Work out the finished part from the listing and answer in its coordinate system (mm). A direction names the side the tool comes from. Give positions to 0.01 mm unless a question says otherwise; leave off trailing zeros. Loops run counter-clockwise (first coordinate to the right, second up) from the corner with the lowest first, then second, coordinate; pieces in that order, holes last.
```python
from build123d import *

# Parameters (mm, degrees)
SKETCH1_W           = 120
SKETCH1_H           = 50
BOSS_EXTRUDE1_DEPTH = 5
SKETCH2_W           = 120
SKETCH2_H           = 50
SKETCH2_W_2         = 117
SKETCH2_H_2         = 47
BOSS_EXTRUDE3_DEPTH = 40
DRAFT2_ANGLE        = 6
FILLET1_R           = 3


with BuildPart() as part:
    # Sketch1 → Boss-Extrude1 (new body)
    with BuildSketch(Plane.XY):
        Rectangle(SKETCH1_W, SKETCH1_H)
    extrude(amount=BOSS_EXTRUDE1_DEPTH)

    # Sketch2 → Boss-Extrude3 (add)
    with BuildSketch(Plane.XY.offset(5)):
        Rectangle(SKETCH2_W, SKETCH2_H)
        Rectangle(SKETCH2_W_2, SKETCH2_H_2, mode=Mode.SUBTRACT)
    extrude(amount=BOSS_EXTRUDE3_DEPTH)

    # Draft2
    draft2_faces = [part.faces().sort_by_distance(p)[0] for p in [
        (-58.5, 0, 25),
        (0, 23.5, 25),
        (58.5, 0, 25),
        (0, -23.5, 25),
    ]]
    draft(draft2_faces, Plane.XY.offset(45), DRAFT2_ANGLE)

    # Fillet1
    fillet1_edges = [part.edges().sort_by_distance(p)[0] for p in [
        (54.295830589, 0, 5),
        (0, 19.295830589, 5),
        (-54.295830589, 0, 5),
        (0, -19.295830589, 5),
        (56.397915295, 21.397915295, 25),
        (-56.397915295, 21.397915295, 25),
        (-56.397915295, -21.397915295, 25),
        (56.397915295, -21.397915295, 25),
    ]]
    fillet(fillet1_edges, radius=FILLET1_R)


solid = part.part
```
Q1. Section B-B on y = -6 is taken. Give the vertices of the cut face in (x, z).
Q2. Consider line 1 along Z through (x, y) = (31, -5); line 2 along Y through (x, z) = (12, 38); line 3 along Y through (x, z) = (10, 42.5). Determine where each line is inside the solid, lowest interval first.
Q3. Section A-A on x = -20.5 is taken. Give the vertices of the cut face in (y, z).
Q4. Determine the mould class of faces 1 (the face through (-60, 0, 22)), 2 (the face through (60, 0, 22)), 3 (the face through (-55.71, -20.67, 26.57)), 4 (the face through (-1, 0, 5)) for opening direction X: +X half, -X half, draft (parallel to the pull), parting line (faces both ways), or undercut.
Q5. Which of the six approach directions +Z, -Z, +X, -X, +Y, -Y give full straight-line access (tool end or side, diameter ignored) to faces 5 (the face through (-0.78, 21.51, 26.08)), 6 (the face through (-1, -25, 22))?
Q6. Given pin 1 (6 mm diameter, centred on x = -32, y = -15, fed in from +Z); pin 2 (10 mm diameter, centred on x = 1.5, y = 3, fed in from +Z), each flat-ended and moving along its own axis, determine where each tip first touches the part or whether it passes through.
Check result:
1. outline: (-60, 0) - (60, 0) - (60, 45) - (58.5, 45) - (54.58, 7.69) arc R3 cw to (51.59, 5) - (-51.59, 5) arc R3 cw to (-54.58, 7.69) - (-58.5, 45) - (-60, 45) - close
2. line 1: z = 0 to 5
2. line 2: y = -25 to -22.76, 22.76 to 25
2. line 3: y = -25 to -23.24, 23.24 to 25
3. outline: (-25, 0) - (25, 0) - (25, 45) - (23.5, 45) - (19.58, 7.69) arc R3 cw to (16.59, 5) - (-16.59, 5) arc R3 cw to (-19.58, 7.69) - (-23.5, 45) - (-25, 45) - close
4. face 1: -X half
4. face 2: +X half
4. face 3: undercut
4. face 4: undercut
5. face 5: +Z
5. face 6: +Z, -Z, +X, -X, -Y
6. pin 1: stops at z = 5.35
6. pin 2: stops at z = 5
